Input: dimensioned drawing with shaded views. Units: mm. Origin: part minimum x, y, z. A direction names the side the tool comes from. Give positions to 0.01 mm unless a question says otherwise; leave off trailing zeros. Loops run counter-clockwise (first coordinate to the right, second up) from the corner with the lowest first, then second, coordinate; pieces in that order, holes last.
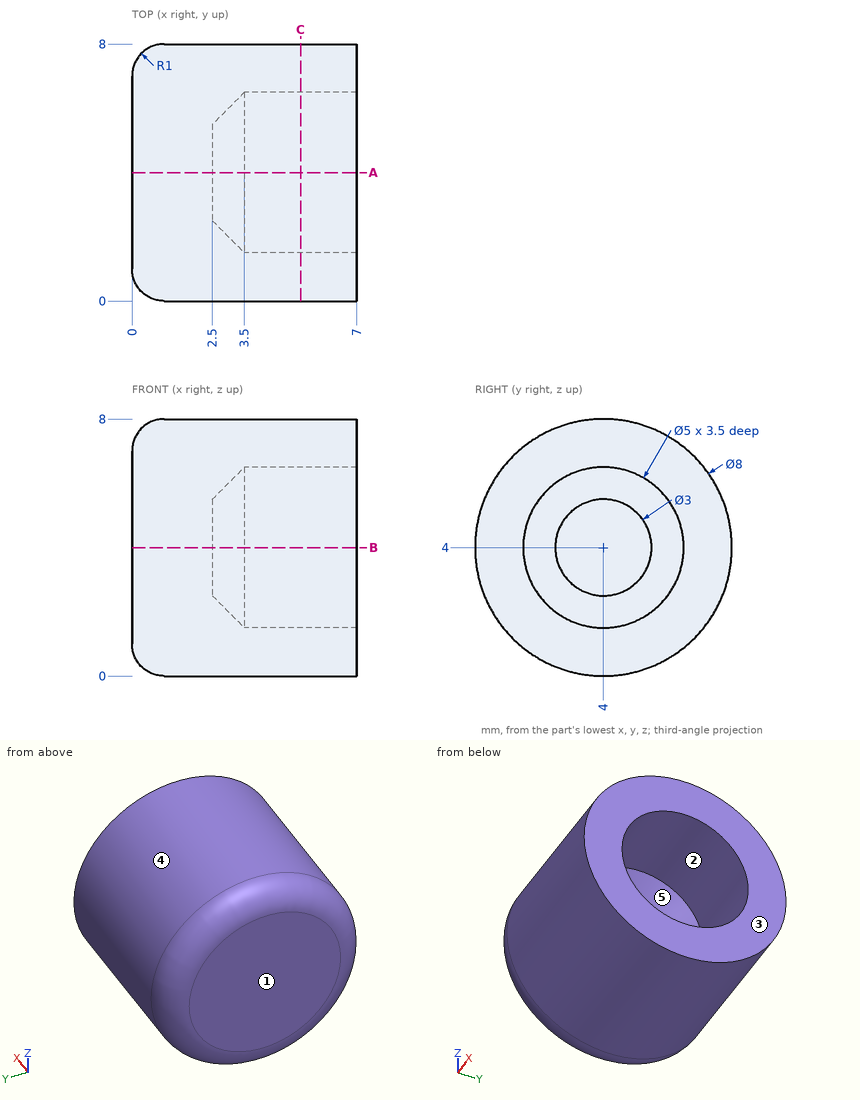
Item 1: Draft query along Y for the marked faces 3, 4 and 5. Return one class per face: +Y half, -Y half, draft (parallel to the pull), parting line (faces both ways), or undercut.
Values follow:
face 3: draft
face 4: parting line
face 5: undercut
Item 2: Section query C-C on x = 5.25. Return loops of the section in (y, z).
Values follow:
outline: circle Ø8 at (4, 4); hole circle Ø5 at (4, 4)
Item 3: Set-up query: the marked faces 1 and 2. Return all of +Z, -Z, +X, -X, +Y, -Y with unobstructed straight access to the full face (end or side cutting, diameter ignored); none if empty.
Values follow:
face 1: +Z, -Z, -X, +Y, -Y
face 2: +X
Item 4: Section query A-A on y = 4. Return loops of the section in (x, z).
Values follow:
outline: (0, 1) arc R1 ccw to (1, 0) - (7, 0) - (7, 1.5) - (3.5, 1.5) - (2.5, 2.5) - (2.5, 5.5) - (3.5, 6.5) - (7, 6.5) - (7, 8) - (1, 8) arc R1 ccw to (0, 7) - close
Item 5: Ray query, probe 1 along Z at (x, y) = (4.9, 4); probe 2 along Z at (x, y) = (4.75, 3.25); probe 3 along Y at (x, z) = (4.75, 4.25). Return the intervals inside material, ascending.
Values follow:
probe 1: z = 0 to 1.5, 6.5 to 8
probe 2: z = 0.07 to 1.62, 6.38 to 7.93
probe 3: y = 0.01 to 1.51, 6.49 to 7.99
Item 6: Pin query (flat end, axial travel): pin 1 (3.5 mm diameter, centred on y = 4, z = 4.5, fed in from +X); pin 2 (1.5 mm diameter, centred on x = 1.5, z = 5.5, fed in from +Y); pin 3 (4 mm diameter, centred on x = 2, z = 1.5, fed in from +Y). Return the tip coordinate at first contact, or that it passes through.
Values follow:
pin 1: stops at x = 3.25
pin 2: stops at y = 7.93
pin 3: stops at y = 7.97
